from build123d import *

# Parameters (mm, degrees)
SKETCH1_R            = 29
SKETCH1_R_2          = 12
BOSS_EXTRUDE1_DEPTH  = 3
SKETCH2_R            = 15
SKETCH2_R_2          = 12
BOSS_EXTRUDE2_DEPTH  = 6
SKETCH3_R            = 15
SKETCH3_R_2          = 10.75
BOSS_EXTRUDE3_DEPTH  = 3
M4_CLEARANCE_HOLE1_D = 4.3
FILLET1_R            = 0.2


with BuildPart() as part:
    # Sketch1 → Boss-Extrude1 (new body)
    with BuildSketch(Plane.XY):
        Circle(SKETCH1_R)
        Circle(SKETCH1_R_2, mode=Mode.SUBTRACT)
    extrude(amount=BOSS_EXTRUDE1_DEPTH)

    # Sketch2 → Boss-Extrude2 (add)
    with BuildSketch(Plane.XY.offset(3)):
        Circle(SKETCH2_R)
        Circle(SKETCH2_R_2, mode=Mode.SUBTRACT)
    extrude(amount=BOSS_EXTRUDE2_DEPTH)

    # Sketch3 → Boss-Extrude3 (add)
    with BuildSketch(Plane.XY.offset(9)):
        Circle(SKETCH3_R)
        Circle(SKETCH3_R_2, mode=Mode.SUBTRACT)
    extrude(amount=-BOSS_EXTRUDE3_DEPTH)

    # M4 Clearance Hole1 (through all)
    with Locations(Plane.XY.offset(3)):
        with Locations((0, 25), (25, 0), (0, -25), (-25, 0), (0, 0)):
            Hole(M4_CLEARANCE_HOLE1_D / 2)

    # Fillet1
    fillet1_edges = [part.edges().sort_by_distance(p)[0] for p in [
        (-15, 0, 3),
        (-12, 0, 6),
    ]]
    fillet(fillet1_edges, radius=FILLET1_R)


solid = part.part
Geometry: final body of the model. Coordinates: model frame, mm. A direction names the side the tool comes from. Give positions to 0.01 mm unless a question says otherwise; leave off trailing zeros. Order: outer loops, then holes, each group sorted by start corner. A loop starts at its lowest first (then second) coordinate and runs counter-clockwise, first axis right, second up. Notation, with made-up numbers: (18, 22) -> (68, 22) arc R13 cw to (68, 44) -> close; hole circle Ø10 at (-19, 54.5). An arc over 180 degrees is marked (long way). Answer as a JSON object with one key per item and string values.
Q1. Section C-C (y = 24). Output: boundary loops of the cut face in (x, z).
Entries:
{"outline": "(-16.28, 0) -> (-1.9, 0) -> (-1.9, 3) -> (-16.28, 3) -> close; (1.9, 0) -> (16.28, 0) -> (16.28, 3) -> (1.9, 3) -> close"}
Q2. Access query for faces 1 (the cylindrical face through (-11.99, 0.53, 2.86)), 2 (the flat face through (12, -12, 3)), 3 (the cylindrical face through (-1.4, 10.66, 7.52)). Directions: +Z, -Z, +X, -X, +Y, -Y. A direction counts if a zero-diameter tool reaches every point of the face in a straight line with its end or side. Return the directions, or none.
Entries:
{"face 1": "-Z", "face 2": "+Z", "face 3": "+Z, -Z"}
Q3. Section B-B (z = 4). Output: boundary loops of the cut face in (x, y), plus the area to 3 significant figures.
Entries:
{"outline": "circle Ø30 at (0, 0); hole circle Ø24 at (0, 0)", "area": "254 mm^2"}
Q4. First-contact query: pin 1 (4 mm diameter, centred on x = -19, y = 18, fed in from +Z); pin 2 (2 mm diameter, centred on x = -12, z = 2.5, fed in from -Y); pin 3 (1.5 mm diameter, centred on x = 16.5, z = 3.5, fed in from +Y); pin 4 (5 mm diameter, centred on x = 9, y = -4, fed in from -Z). Flat tips, straight axial feed; report the tip coordinate or a pass-through.
Entries:
{"pin 1": "stops at z = 3", "pin 2": "stops at y = -26.83", "pin 3": "stops at y = 24.23", "pin 4": "stops at z = 0"}
Q5. Section A-A (x = 0). Output: boundary loops of the cut face in (y, z), plus the area to 3 significant figures.
Entries:
{"outline": "(-29, 0) -> (-27.15, 0) -> (-27.15, 3) -> (-29, 3) -> close; (-22.85, 0) -> (-12, 0) -> (-12, 5.8) arc R0.2 cw to (-11.8, 6) -> (-10.75, 6) -> (-10.75, 9) -> (-15, 9) -> (-15, 3.2) arc R0.2 cw to (-15.2, 3) -> (-22.85, 3) -> close; (10.75, 6) -> (11.8, 6) arc R0.2 cw to (12, 5.8) -> (12, 0) -> (22.85, 0) -> (22.85, 3) -> (15.2, 3) arc R0.2 cw to (15, 3.2) -> (15, 9) -> (10.75, 9) -> close; (27.15, 0) -> (29, 0) -> (29, 3) -> (27.15, 3) -> close", "area": "120 mm^2"}
Q6. Draft query along Y for faces 4 (the cylindrical face through (-14.985, 0.66, 6.059)), 5 (the cylindrical face through (-27.05, 0.65, 1.48)), 6 (the cylindrical face through (22.95, 0.65, 1.48)), 7 (the flat face through (12.5, 0.4, 0)). Return one class per face: released by +Y, released by -Y, zero draft, split by the parting line, or undercut.
Entries:
{"face 4": "split by the parting line", "face 5": "undercut", "face 6": "undercut", "face 7": "zero draft"}
Q7. Material intervals for probe 1 along Y at (x, z) = (1, 1.5); probe 2 along Z at (x, y) = (-6.5, 23); probe 3 along Y at (x, z) = (-3.5, 7.5), sorted ascending.
Entries:
{"probe 1": "y = -28.98 to -26.9, -23.1 to -11.96, 11.96 to 23.1, 26.9 to 28.98", "probe 2": "z = 0 to 3", "probe 3": "y = -14.59 to -10.16, 10.16 to 14.59"}
